Source: CAD feature listing. Evaluate the final solid. Frame: model axes, mm. Face numbers are marked on the shaded views. A direction names the side the tool comes from. Round coordinates to 2 decimals unless told otherwise and drop trailing zeros. Order: outer loops, then holes, each group sorted by start corner. A loop starts at its lowest first (then second) coordinate and runs counter-clockwise, first axis right, second up. Notation, with made-up numbers: (7, 22.5) - (50, 22.5) arc R19 ccw to (50, 47.5) - close; hole circle Ø9 at (34, 63.5). An arc over 180 degrees is marked (long way). Put each result on its own line as item: value. Start each with the question number.
1) Section A-A on y = 0. Output: boundary loops of the cut face in (x, z), then the cut area to 3 significant figures.
2) Line query: probe 1 along Y at (x, z) = (0, 0.8); probe 2 along X at (y, z) = (3, 0.6); probe 3 along X at (y, z) = (-0.25, 2.5). Output: solid intervals per line, ascending. Write a range as [from, to].
3) Access query for the marked faces 4, 5 and 6. Directions: +Z, -Z, +X, -X, +Y, -Y. A direction counts if a zero-diameter tool reaches every point of the face in a straight line with its end or side. Return the directions, or none.
4) Section B-B on z = 0.7. Output: boundary loops of the cut face in (x, y), then the cut area to 3 significant figures.
5) Contact query for flat-ended pins moving along their axis: P1, Ø4, axis at x = -28, y = 0.5, coming from the +Z side; P2, Ø2.5, axis at x = -0.5, y = 0.5, coming from the -Z side; P3, Ø2, axis at x = -1, y = 4.5, coming from the -Z side. Output: stop coordinate, or through.
6) Section C-C on x = -2.5. Output: boundary loops of the cut face in (y, z), then the cut area to 3 significant figures.
7) Section D-D on y = -4.5. Output: boundary loops of the cut face in (x, z).
8) Mould query, pull axis X, two halves, no side actions, for the marked faces 1, 2 and 3. Classes: +X half, -X half, draft (parallel to the pull), parting line (faces both ways), or undercut.
```python
from build123d import *

# Parameters (mm, degrees)
EXTRUDE_1_DEPTH          = 6
SKETCH_3_R               = 4.1
CUT_EXTRUDE_2_DEPTH      = 1.2
SKETCH_4_R               = 4.1
CUT_EXTRUDE_3_DEPTH      = 4
SKETCH_5_R               = 3.5
CUT_EXTRUDE_5_DEPTH      = 37.986484018
CUT_EXTRUDE_6_DEPTH      = 37.986484018
CUT_EXTRUDE_6_DEPTH_BACK = 37.986484018
SKETCH_6_R               = 1.9


with BuildPart() as part:
    # ｽｹｯﾁ1 → ﾎﾞｽ - 押し出し1 (new body)
    with BuildSketch(Plane.XY):
        with BuildLine():
            Line((0.166666667, 4.99722145), (-29.8, 5.99666574))
            ThreePointArc((-29.8, 5.99666574), (-36, 0), (-29.8, -5.99666574))
            Line((-29.8, -5.99666574), (0.166666667, -4.99722145))
            ThreePointArc((0.166666667, -4.99722145), (5, 0), (0.166666667, 4.99722145))
        make_face()
    extrude(amount=EXTRUDE_1_DEPTH)

    # ｽｹｯﾁ3 → ｶｯﾄ - 押し出し2 (cut)
    with BuildSketch(Plane(origin=(0, 0, 0), x_dir=(-1, 0, 0), z_dir=(0, 0, -1))):
        Circle(SKETCH_3_R)
    extrude(amount=-CUT_EXTRUDE_2_DEPTH, mode=Mode.SUBTRACT)

    # ｽｹｯﾁ4 → ｶｯﾄ - 押し出し3 (cut)
    with BuildSketch(Plane.XY.offset(6)):
        with Locations((-30, 0)):
            Circle(SKETCH_4_R)
    extrude(amount=-CUT_EXTRUDE_3_DEPTH, mode=Mode.SUBTRACT)

    # ｽｹｯﾁ5 → ｶｯﾄ - 押し出し5 (cut, through all)
    with BuildSketch(Plane.XY.offset(6)):
        with Locations((-30, 0)):
            Circle(SKETCH_5_R)
    extrude(amount=-CUT_EXTRUDE_5_DEPTH, mode=Mode.SUBTRACT)

    # ｽｹｯﾁ6 → ｶｯﾄ - 押し出し6 (cut, two sides: drawn at the far end of the back side and taken through both)
    with BuildSketch(Plane.XY.offset(6).offset(-CUT_EXTRUDE_6_DEPTH_BACK)):
        with Locations(Location((0, 0, 0), (0, 0, 180))):
            Circle(SKETCH_6_R)
    extrude(amount=CUT_EXTRUDE_6_DEPTH + CUT_EXTRUDE_6_DEPTH_BACK, mode=Mode.SUBTRACT)


solid = part.part
```
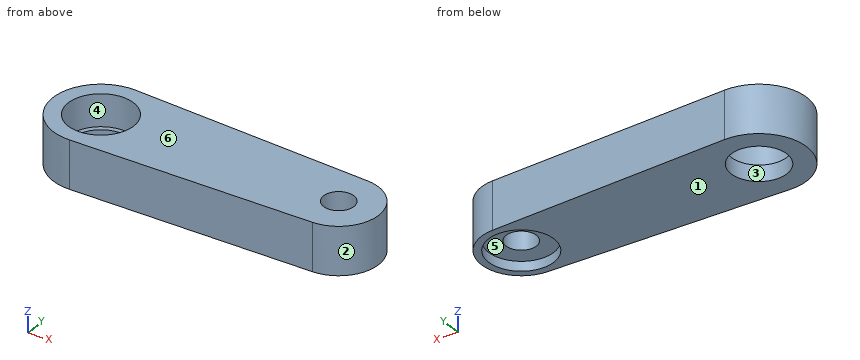
Answer sheet:
1. outline: (-36, 0) - (-33.5, 0) - (-33.5, 2) - (-34.1, 2) - (-34.1, 6) - (-36, 6) - close; (-26.5, 0) - (-4.1, 0) - (-4.1, 1.2) - (-1.9, 1.2) - (-1.9, 6) - (-25.9, 6) - (-25.9, 2) - (-26.5, 2) - close; (1.9, 1.2) - (4.1, 1.2) - (4.1, 0) - (5, 0) - (5, 6) - (1.9, 6) - close
1. area: 171 mm^2
2. probe 1: [-5, -4.1], [4.1, 5]
2. probe 2: [-35.2, -31.8], [-28.2, -2.79], [2.79, 4]
2. probe 3: [-35.99, -34.09], [-25.91, -1.88], [1.88, 4.99]
3. face 4: +Z
3. face 5: -Z
3. face 6: +Z, +X, -X, +Y, -Y
4. outline: (-29.8, -6) - (0.17, -5) arc R5 ccw to (0.17, 5) - (-29.8, 6) arc R6 ccw (long way) to start; hole circle Ø7 at (-30, 0); hole circle Ø8.2 at (0, 0)
4. area: 335 mm^2
5. P1: z = 2
5. P2: z = 1.2
5. P3: z = 0
6. outline: (-5.09, 0) - (-3.25, 0) - (-3.25, 1.2) - (3.25, 1.2) - (3.25, 0) - (5.09, 0) - (5.09, 6) - (-5.09, 6) - close
6. area: 53.2 mm^2
7. outline: (-33.97, 0) - (2.18, 0) - (2.18, 6) - (-33.97, 6) - close
8. face 1: draft
8. face 2: +X half
8. face 3: undercut
